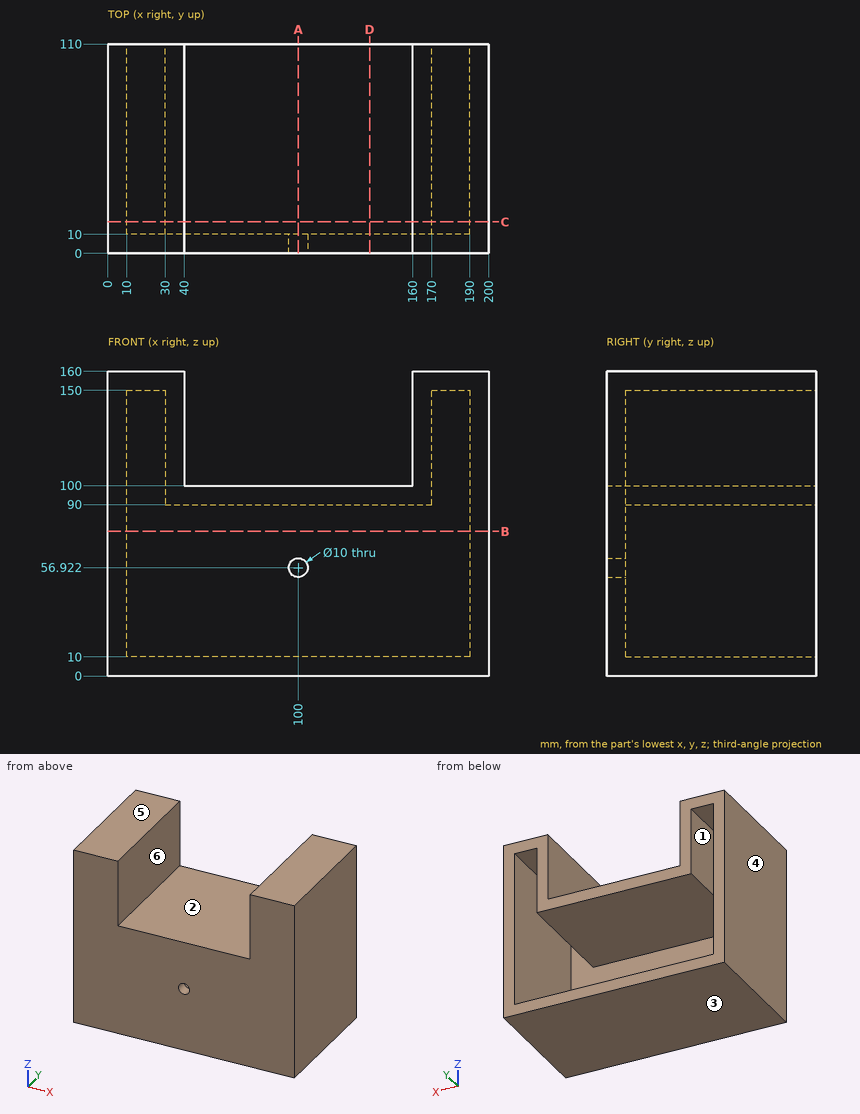
Study the drawing (mm; zero at the part's minimum x, y, z) and answer. A direction names the side the tool comes from. Coordinates: 2 decimals unless noted, no trailing zeros. Loops run counter-clockwise (first coordinate to the right, second up) from the corner with the lowest first, then second, coordinate; pieces in that order, holes last. Notation, with made-up numbers: (74, -39) -> (99, -39) arc R24 cw to (99, -17) -> close; hole circle Ø2 at (-2.5, 8). An arc over 180 degrees is marked (long way). Write each question's results on one line, items separated by ' | '. Start each with the question number.
1) Consider line 1 along X through (y, z) = (30, 143); line 2 along X through (y, z) = (24.5, 98.5); line 3 along Z through (x, y) = (100, 4). Determine where each line is inside the solid, lowest interval first.
2) Find section A-A on x = 100. Determine the outline of the cut face in (y, z), then the cut area to 3 significant figures.
3) The mould has two halves that part along X. Classify the marked faces 4, 5 and 6: pulls with the +X half, pulls with the -X half, needs draft (parallel to the pull), parting line crosses it, or undercut.
4) For the marked faces 1, 2 and 3, determine the directions among +Z, -Z, +X, -X, +Y, -Y from which every point of the face is accessible in a straight line to the end or side of a thin tool.
5) Flat-ended cylindrical pins translate along their axes: P1, Ø2, axis at x = 134.5, y = 83, coming from the +Z side; P2, Ø6, axis at x = 100, z = 56.92, coming from the +Y side; P3, Ø2, axis at x = 107, z = 46.5, coming from the +Y side. Find the tip coordinate at first contact, or state that the pin passes through.
6) Find section C-C on y = 16.5. Determine the outline of the cut face in (x, z), then the cut area to 3 significant figures.
7) Find section B-B on z = 76. Determine the outline of the cut face in (x, y), then the cut area to 3 significant figures.
8) Find section D-D on x = 137.5. Determine the outline of the cut face in (y, z).
Response values:
1) line 1: x = 0 to 10, 30 to 40, 160 to 170, 190 to 200 | line 2: x = 0 to 10, 30 to 170, 190 to 200 | line 3: z = 0 to 51.92, 61.92 to 100
2) outline: (0, 0) -> (110, 0) -> (110, 10) -> (10, 10) -> (10, 51.92) -> (0, 51.92) -> close; (0, 61.92) -> (10, 61.92) -> (10, 90) -> (110, 90) -> (110, 100) -> (0, 100) -> close | area: 2,900 mm^2
3) face 4: pulls with the -X half | face 5: needs draft | face 6: undercut
4) face 1: +Y | face 2: +Z, +Y, -Y | face 3: -Z, +X, -X, +Y, -Y
5) P1: stops at z = 100 | P2: passes through | P3: stops at y = 10
6) outline: (0, 0) -> (200, 0) -> (200, 160) -> (160, 160) -> (160, 100) -> (40, 100) -> (40, 160) -> (0, 160) -> close; hole (10, 10) -> (190, 10) -> (190, 150) -> (170, 150) -> (170, 90) -> (30, 90) -> (30, 150) -> (10, 150) -> close | area: 8,000 mm^2
7) outline: (0, 0) -> (200, 0) -> (200, 110) -> (190, 110) -> (190, 10) -> (10, 10) -> (10, 110) -> (0, 110) -> close | area: 4,000 mm^2
8) outline: (0, 0) -> (110, 0) -> (110, 10) -> (10, 10) -> (10, 90) -> (110, 90) -> (110, 100) -> (0, 100) -> close
